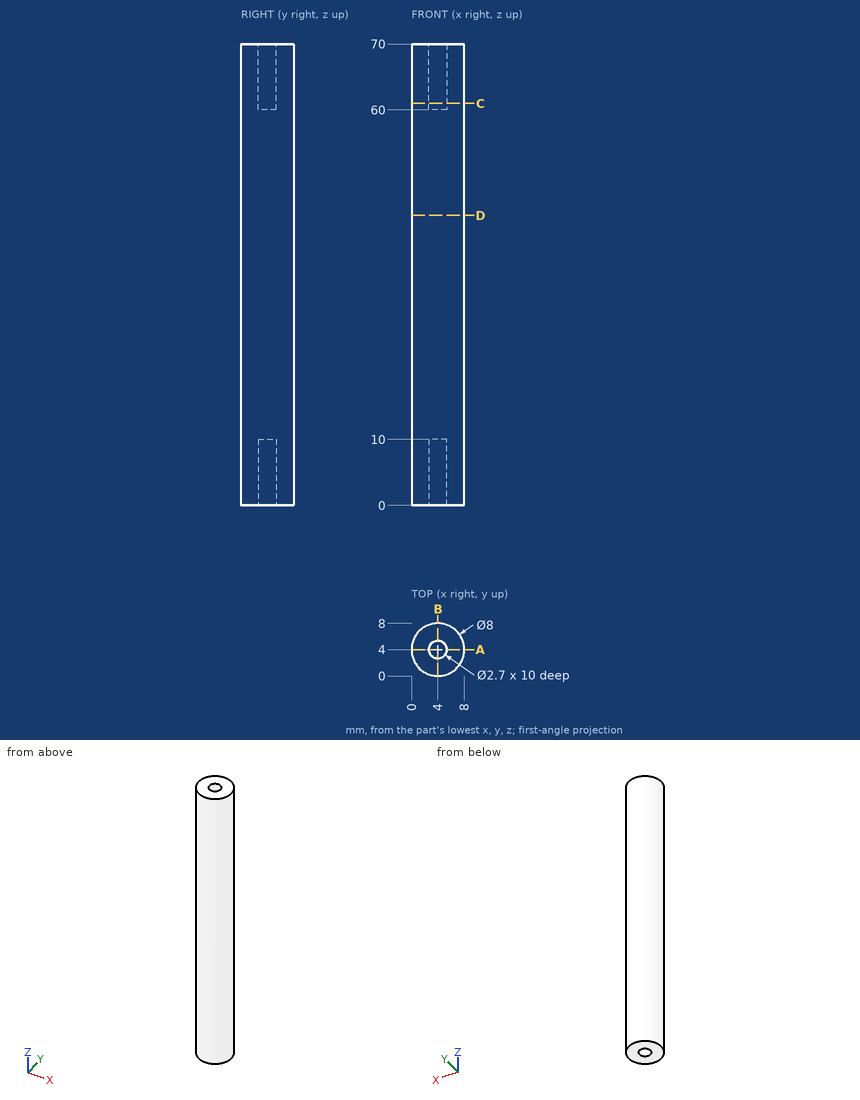
Verification items for this drawing (mm, ordinates from the low corner). Give positions to 0.01 mm unless a question says otherwise; leave off trailing zeros. Loops run counter-clockwise (first coordinate to the right, second up) from the corner with the lowest first, then second, coordinate; pieces in that order, holes last. Notation, with made-up numbers: M 56,-28.75 L 69,-28.75 A38 ccw 69,9.25 Z; hole C 52.5,39.25 d2. An arc over 180 degrees is marked long. Answer as a JSON object with one key per item and string values. Group by question number.
Q1. Cross-section at C-C on z = 61. Record the cut outline in (x, y).
Q2. Cross-section at D-D on z = 44. Record the cut outline in (x, y).
Q3. Material ranges on line 1 along Y through (x, z) = (4, 7.5); line 2 along Y through (x, z) = (4.25, 17), recorded low to high. Write a range as [from, to].
Q4. Cross-section at A-A on y = 4. Record the cut outline in (x, z).
Q5. Go/stop test with flat-tipped pins: P1, Ø3, axis at x = 4, y = 4.5, coming from the +Z side; P2, Ø1, axis at y = 1.5, z = 26.5, coming from the -X side; P3, Ø1.5, axis at y = 1.5, z = 21, coming from the -X side; P4, Ø2, axis at x = 4, y = 4, coming from the -Z side. Record where each tip stops, or that it passes through.
Evaluation:
{
 "1": {"outline": "C 4,4 d8; hole C 4,4 d2.7"},
 "2": {"outline": "C 4,4 d8"},
 "3": {"line 1": "y = [0, 2.65], [5.35, 8]", "line 2": "y = [0.01, 7.99]"},
 "4": {"outline": "M 0,0 L 2.65,0 L 2.65,10 L 5.35,10 L 5.35,0 L 8,0 L 8,70 L 5.35,70 L 5.35,60 L 2.65,60 L 2.65,70 L 0,70 Z"},
 "5": {"P1": "stops at z = 70", "P2": "stops at x = 0.54", "P3": "stops at x = 0.4", "P4": "stops at z = 10"}
}
